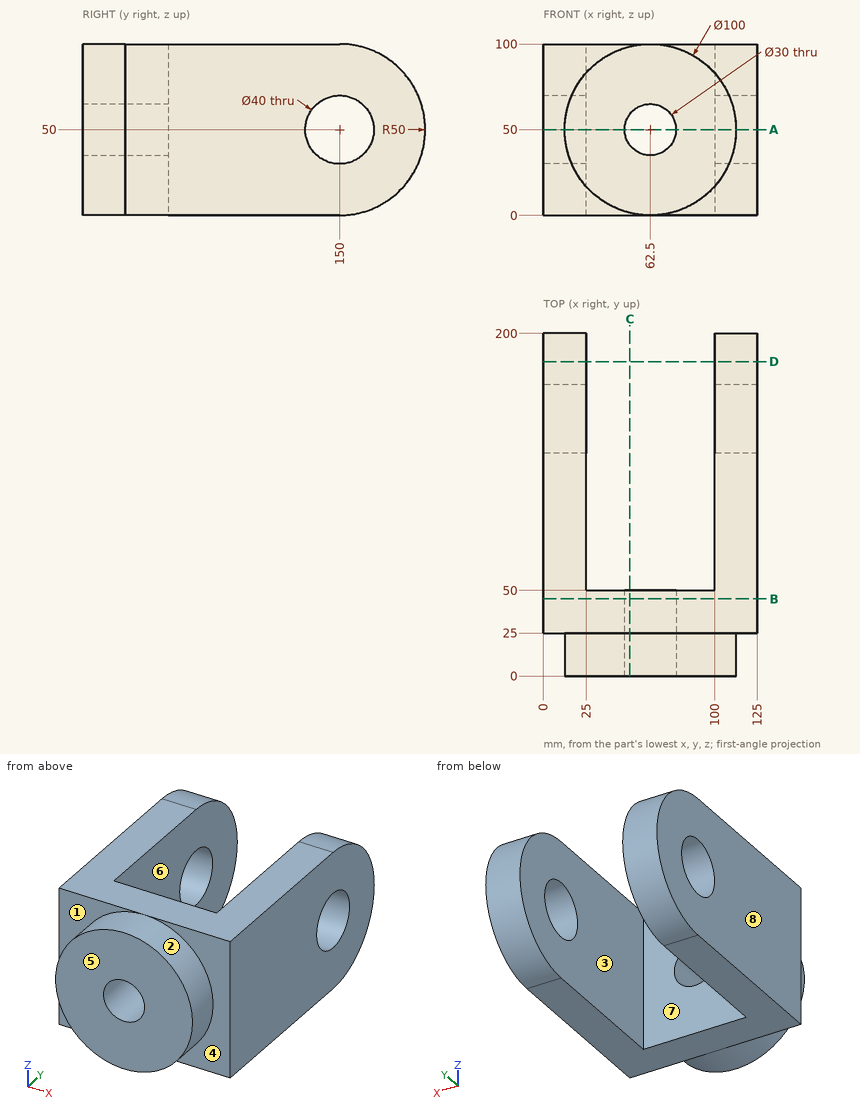
Could you check a few things on this drawing? It's one solid part, dimensions in mm from its lowest x, y, z. A direction names the side the tool comes from. Round coordinates to 2 decimals unless told otherwise and drop trailing zeros. Write each loop counter-clockwise with the first axis right and the second up, starting at its lowest first coordinate (ties: lowest second). Pieces come first, ordered by that corner, then holes.
Q1. If we section it at A-A on z = 50: Write out the boundary of the cut face in (x, y).
Q2. If we section it at C-C on x = 50.5: Write out the boundary of the cut face in (y, z).
Q3. If we mould it in two halves opening along X, with no side actions, what happens to the marked faces 5, 6, 7 and 8? For each: +X half, -X half, draft (parallel to the pull), parting line (faces both ways), or undercut.
Q4. Which directions (+Z, -Z, +X, -X, +Y, -Y) give clear straight access to the entire face, cutting with the end or side of a thin tool? Please do the marked faces 1, 2, 3 and 4.
Q5. If we section it at D-D on y = 183.5: Write out the boundary of the cut face in (x, z), plus the area to 3 significant figures.
Q6. If we section it at B-B on y = 45: Write out the boundary of the cut face in (x, z).
Q7. Will this pin go through, and if not, where does the flat tip stop? P1, Ø22.5, axis at x = 60.5, z = 72, coming from the +Y side.
Q8. Please list where these lines run through material, in increasing order: probe 1 along Y at (x, z) = (105, 50); probe 2 along X at (y, z) = (168, 12.5); probe 3 along Y at (x, z) = (12, 50).
Answer below:
1. outline: (0, 25) - (12.5, 25) - (12.5, 0) - (47.5, 0) - (47.5, 50) - (25, 50) - (25, 130) - (0, 130) - close; (0, 170) - (25, 170) - (25, 200) - (0, 200) - close; (77.5, 0) - (112.5, 0) - (112.5, 25) - (125, 25) - (125, 130) - (100, 130) - (100, 50) - (77.5, 50) - close; (100, 170) - (125, 170) - (125, 200) - (100, 200) - close
2. outline: (0, 1.46) - (25, 1.46) - (25, 0) - (50, 0) - (50, 41) - (0, 41) - close; (0, 59) - (50, 59) - (50, 100) - (25, 100) - (25, 98.54) - (0, 98.54) - close
3. face 5: draft
3. face 6: undercut
3. face 7: undercut
3. face 8: -X half
4. face 1: -X, -Y
4. face 2: -Y
4. face 3: +Z, -Z, +Y
4. face 4: +X, -Y
5. outline: (0, 12.88) - (25, 12.88) - (25, 87.12) - (0, 87.12) - close; (100, 12.88) - (125, 12.88) - (125, 87.12) - (100, 87.12) - close
5. area: 3,710 mm2
6. outline: (0, 0) - (125, 0) - (125, 100) - (0, 100) - close; hole circle Ø30 at (62.5, 50)
7. P1: stops at y = 50
8. probe 1: y = 0 to 130, 170 to 200
8. probe 2: x = 0 to 25, 100 to 125
8. probe 3: y = 25 to 130, 170 to 200
